The listing builds one solid part. Answer for the finished solid, in the listing's coordinates (mm). Face numbers are marked on the shaded views. A direction names the side the tool comes from. Coordinates: 2 decimals unless noted, no trailing zeros. Order: outer loops, then holes, each group sorted by start corner. A loop starts at its lowest first (then second) coordinate and runs counter-clockwise, first axis right, second up.
```python
from build123d import *

# Parameters (mm, degrees)
SZKIC1_R                    = 10
DODANIE_WYCI_GNI_CIE1_DEPTH = 5
ZAOKR_GLENIE3_R             = 2
SZKIC2_R                    = 15
DODANIE_WYCI_GNI_CIE2_DEPTH = 5


with BuildPart() as part:
    # Szkic1 → Dodanie-wyciągnięcie1 (new body)
    with BuildSketch(Plane(origin=(0, 0, 0), x_dir=(1, 0, 0), z_dir=(0, 1, 0))):
        with Locations(Location((0, 0, 0), (0, 0, 270))):
            Circle(SZKIC1_R)
    extrude(amount=DODANIE_WYCI_GNI_CIE1_DEPTH)

    # Zaokrąglenie3
    zaokr_glenie3_edges = [part.edges().sort_by_distance(p)[0] for p in [
        (0, 0, -10),
    ]]
    fillet(zaokr_glenie3_edges, radius=ZAOKR_GLENIE3_R)

    # Szkic2 → Dodanie-wyciągnięcie2 (add)
    with BuildSketch(Plane(origin=(0, 5, 0), x_dir=(1, 0, 0), z_dir=(0, 1, 0))):
        with Locations(Location((0, 0, 0), (0, 0, 270))):
            Circle(SZKIC2_R)
    extrude(amount=DODANIE_WYCI_GNI_CIE2_DEPTH)


solid = part.part
```
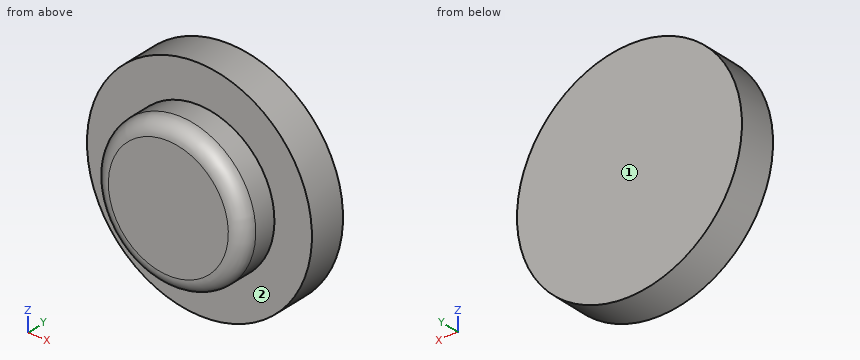
1) For the marked faces 1 and 2, determine the directions among +Z, -Z, +X, -X, +Y, -Y from which every point of the face is accessible in a straight line to the end or side of a thin tool.
2) A cutting plane is placed at B-B, the plane x = 0. Write down the section's boundary in (y, z).
3) A cutting plane is placed at C-C, the plane y = 6.25. Write down the section's boundary in (x, z).
4) Straight lines are drawn through the part: probe 1 along Y at (x, z) = (9.75, 11); probe 2 along X at (y, z) = (6.5, 0); probe 3 along Z at (x, y) = (-2.75, 7.75). For each, find the intervals that lie inside material, in ascending order.
5) A cutting plane is placed at A-A, the plane z = 0. Write down the section's boundary in (x, y), plus the area to 3 significant figures.
6) Each of these flat-tipped pins is pushed along its axis until it touches: P1, Ø1, axis at x = 10, z = 1, coming from the -Y side; P2, Ø9, axis at x = 3, z = -2.5, coming from the -Y side; P3, Ø3, axis at y = 8, z = 10.5, coming from the -X side; P4, Ø1.5, axis at x = 2, y = 6.5, coming from the -Z side. Where does it stop, or does it pass through?
7) A cutting plane is placed at D-D, the plane y = 2.5. Write down the section's boundary in (x, z).
Working result:
1. face 1: +Z, -Z, +X, -X, +Y
1. face 2: -Y
2. outline: (0, -8) arc R2 ccw to (2, -10) - (5, -10) - (5, -15) - (10, -15) - (10, 15) - (5, 15) - (5, 10) - (2, 10) arc R2 ccw to (0, 8) - close
3. outline: circle Ø30 at (0, 0)
4. probe 1: y = 5 to 10
4. probe 2: x = -15 to 15
4. probe 3: z = -14.75 to 14.75
5. outline: (-15, 5) - (-10, 5) - (-10, 2) arc R2 ccw to (-8, 0) - (8, 0) arc R2 ccw to (10, 2) - (10, 5) - (15, 5) - (15, 10) - (-15, 10) - close
5. area: 248 mm2
6. P1: stops at y = 0.74
6. P2: stops at y = 0
6. P3: stops at x = -12
6. P4: stops at z = -14.95
7. outline: circle Ø20 at (0, 0)
